Verification items for the finished model (mm, model axes). A direction names the side the tool comes from. Round coordinates to 2 decimals unless told otherwise and drop trailing zeros. Order: outer loops, then holes, each group sorted by start corner. A loop starts at its lowest first (then second) coordinate and runs counter-clockwise, first axis right, second up. Notation, with made-up numbers: (-31.75, -21.75) -> (-13.75, -21.75) arc R10 ccw to (-13.75, -16.75) -> close; hole circle Ø9 at (16, 18). An arc over 180 degrees is marked (long way). Put each result on its own line as item: value.
Autodesk Inventor part; units mm, degrees
ref_plane "Work Plane1" through (29, 0, 0) normal (0, -1, 0) x (1, 0, 0)
ref_plane "YZ Plane" through (0, 0, 0) normal (1, 0, 0) x (0, 1, 0)
ref_plane "XZ Plane" through (0, 0, 0) normal (0, 1, 0) x (-1, 0, 0)
sketch "스케치1" plane through (0, 0, 0) normal (0, 0, 1) x (1, 0, 0)
  line L0 (-2.3333, 0) -> (25, 0)
  line L1 (25, 0) -> (25, 5)
  line L2 (25, 5) -> (3.75, 5)
  line L3 (3.75, 5) -> (2.8297, 5)
  line L4 (2.8297, 5) -> (0, 5)
  line L5 (0, 5) -> (0, 8)
  line L6 (0, 8) -> (-10, 8)
  line L7 (-10, 8) -> (-10, 4.6188)
  line L8 (-10, 4.6188) -> (-5, 4.6188)
  line L9 (-5, 4.6188) -> (-2.3333, 0)
  line L10 (-17, 0) -> (32, 0)
  line L11 (0, -1.6) -> (0, 9.6)
  line L12 (3.75, 5) -> (0, 5) construction
  dimension "d1" = 21.25
  dimension "d2" = 0.9203
  dimension "d3" = 10
  dimension "d4" = 5
  dimension "d5" = 60
  dimension "d6" = 10
  dimension "d7" = 10
  dimension "d8" = 9.2376
  dimension "d9" = 16
  dimension "d26" = 25
revolve "본체" add sketch "스케치1" angle 360 about axis through (-2.3333, 0, 0) along (1, 0, 0)
sketch "스케치2" plane through (-10, 0, 0) normal (-1, 0, 0) x (0, 0, 1)
  circle A0 centre (0, 0) radius 4.6188
  line L0 (0, -11.2) -> (0, 11.2)
  line L1 (-11.2, 0) -> (11.2, 0)
  line L2 (4.6188, 0) -> (2.3094, -4)
  line L3 (2.3094, -4) -> (-2.3094, -4)
  line L4 (-2.3094, -4) -> (-4.6188, 0)
  line L5 (-4.6188, 0) -> (-2.3094, 4)
  line L6 (-2.3094, 4) -> (2.3094, 4)
  line L7 (2.3094, 4) -> (4.6188, 0)
  point P0 (0, 0)
extrude "슬롯" add sketch "스케치2" against normal up to next contours L7 A0 | A0 L2 | L6 L0 A0 | A0 L0 L3 | L0 L6 A0 | A0 L3 L0 | L4 A0 | A0 L5
fillet "모깎기1" radius 1 1 edges at (-10, -8, 0)
thread "스레드"
chamfer "모따기1" distance 0.9202 distance2 0.9202 1 edges at (25, -5, 0) measured on face at (25, -0.8193, -0.3214)
ref_plane "Work Plane1" through (29, 0, 0) normal (0, -1, 0) x (1, 0, 0)
fillet "Fillet2" radius 0.1 1 edges at (0, -5, 0)
equation "\"d1\" = GEL"
equation "\"d3\" = KOH"
equation "\"d4\" = INTI"
equation "\"d6\" = GD"
equation "\"d7\" = BDM"
equation "\"d8\" = 1.1547 * SW"
equation "\"d9\" = KOD"
equation "\"d26\" = NLG"
equation "\"d30\" = R"
equation "\"d17\" = RR"
equation "\"d13\" = GEL"
equation "\"d15\" = -0.5 * SPD + 0.5 * GD"
equation "\"d16\" = GUL"
equation "\"GD\" = 10"
equation "\"NLG\" = 25"
equation "\"GEL\" = 21.25"
equation "\"KOD\" = 16"
equation "\"KOH\" = 10"
equation "\"INTI\" = 5"
equation "\"GAL\" = 0.61345 * PTC"
equation "\"GUL\" = 0.61345 * PTC"
equation "\"BDM\" = NND"
equation "\"SW\" = 8"
equation "\"RR\" = 1"
equation "\"SPD\" = NND - 1.2269 * PTC"
equation "\"R\" = 0.1"
equation "\"TOA\" = 30deg"
equation "\"GD1\" = THREADDIA - 1.2269 * PTC"
equation "\"FAWI\" = 45deg"
equation "\"PTC\" = 1.5"
equation "\"E0\" = 1.155 * SW"
properties part number "ISO 4762 - M10 x 25(1)" material "스테인레스 스틸, 440C"
Item 1: Material ranges on L1, parallel to X at y = -6.5, z = -1; L2, parallel to Y at x = 10, z = 3; L3, parallel to Y at x = -8, z = -1.5, recorded low to high. Write a range as [from, to].
Check sheet entries:
L1: x = [-10, 0]
L2: y = [-4, 4]
L3: y = [-7.86, -4], [4, 7.86]
Item 2: Tool access check on faces 4 (the cylindrical face through (11.92, -1.08, 4.88)), 5 (the flat face through (-7.36, 1.97, -3.48)), 6 (the flat face through (-10, -5, 0)). Record the directions out of +Z, -Z, +X, -X, +Y, -Y that give a thin tool (end or side, any length) a straight path to the whole face; none if there is none.
Check sheet entries:
face 4: +X
face 5: -X
face 6: +Z, -Z, -X, +Y, -Y
Item 3: Release check for a two-part mould opening along Y. For faces 1 (the flat face through (25, 0, 0)), 2 (the flat face through (-7, 4, 0)), 3 (the cylindrical face through (-4.56, -1.73, 7.81)) record: +Y half, -Y half, draft (parallel to the pull), parting line (faces both ways), or undercut.
Check sheet entries:
face 1: draft
face 2: undercut
face 3: parting line
Item 4: Section check B-B on x = 22. Record the boundary of the cut face in (y, z).
Check sheet entries:
outline: circle Ø10 at (0, 0)
Item 5: Section check A-A on x = -0.5. Record the boundary of the cut face in (y, z).
Check sheet entries:
outline: circle Ø16 at (0, 0)
Item 6: Gauge pin test, flat ends, axial feed: pin 1 Ø4 at (x, z) = (17.5, -2.5) entering from +Y; pin 2 Ø1.4 at (x, z) = (-8, 1) entering from +Y; pin 3 Ø2 at (x, z) = (-1, 2) entering from +Y. Record the tip position at first contact, or that the pin passes through.
Check sheet entries:
pin 1: stops at y = 4.97
pin 2: stops at y = 7.99
pin 3: stops at y = 7.94
